Can you work these out from the model? Positions are in its coordinate system, mm. Give positions to 0.01 mm unless a question says otherwise; leave off trailing zeros. Order: outer loops, then holes, each group sorted by start corner. A loop starts at its lowest first (then second) coordinate and runs counter-clockwise, first axis right, second up. Notation, with made-up numbers: (48.5, 33.25) - (96.5, 33.25) arc R17 ccw to (96.5, 48.25) - close; hole circle Ø8 at (17.25, 11.25). An arc over 180 degrees is marked (long way). Answer as a JSON object with one key per item and string values.
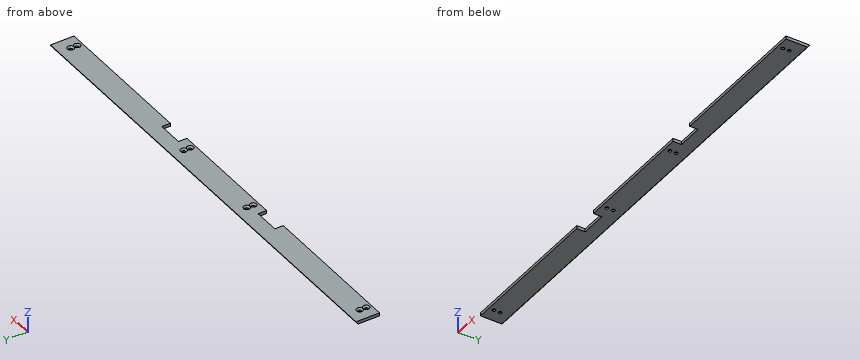
```python
from build123d import *

# Parameters (mm, degrees)
F0_W           = 1840
F0_H           = 92
F1_DEPTH       = 6
F2_W           = 100
F2_H           = 33
F3_DEPTH       = 12.001
F5_DEPTH       = 1840.001
F7_D           = 13
F7_CSINK_D     = 25
F7_CSINK_ANGLE = 90


with BuildPart() as f1:
    # F0 (on Top) → F1 (new body, symmetric)
    with BuildSketch(Plane.XY):
        Rectangle(F0_W, F0_H)
    extrude(amount=F1_DEPTH, both=True)

    # F2 (on face) → F3 (cut, through all)
    with BuildSketch(Plane.XY.offset(6)):
        with Locations((-290, -29.5)):
            Rectangle(F2_W, F2_H)
        with Locations((290, -29.5)):
            Rectangle(F2_W, F2_H)
    extrude(amount=-F3_DEPTH, mode=Mode.SUBTRACT)

    # F4 (on face) → F5 (cut, through all)
    with BuildSketch(Plane.YZ.offset(920)):
        Polygon((46, -6), (46, 4), (37.609004, -6), align=None)
    extrude(amount=-F5_DEPTH, mode=Mode.SUBTRACT)

    # F7 (through all)
    with Locations(Plane.XY.offset(6)):
        with Locations((-870, -1), (-870, -26), (-190, -1), (-190, -26), (190, -26), (190, -1), (870, -1), (870, -26)):
            CounterSinkHole(F7_D / 2, F7_CSINK_D / 2, counter_sink_angle=F7_CSINK_ANGLE)


solid = f1.part
```
Q1. I need wall thicknesses on L1, parallel to X at y = -40.5, z = 2.5; L2, parallel to X at y = -1, z = -4.4; L3, parallel to Y at x = 190, z = -2.45. Which ranges of each line are inside material? Lowest first, please.
Recorded:
{"L1": "x = -920 to -340, -240 to 240, 340 to 920", "L2": "x = -920 to -876.5, -863.5 to -196.5, -183.5 to 183.5, 196.5 to 863.5, 876.5 to 920", "L3": "y = -46 to -32.5, -19.5 to -7.5, 5.5 to 40.59"}
Q2. I'm going to push flat-ended pins straight in: pin 1 Ø10.5 at (x, y) = (-870, -1) entering from +Z; pin 2 Ø1.5 at (x, z) = (-132, 3.5) entering from +Y; pin 3 Ø3.5 at (x, z) = (269, -2) entering from -Y. Where does each tip first touch, or does it pass through?
Recorded:
{"pin 1": "passes through", "pin 2": "stops at y = 46", "pin 3": "stops at y = -13"}
Q3. If we section it at A-A, the plane z = -3.5: Count the separate pieces of the cut face and the enclosed holes in it, then the cut area to 3 significant figures.
Recorded:
{"separate pieces": "1", "enclosed holes": "8", "area": "150,000 mm^2"}
Q4. If we section it at B-B, the plane x = -322: Please give me the cut outline in (y, z), then the cut area to 3 significant figures.
Recorded:
{"outline": "(-13, -6) - (37.61, -6) - (46, 4) - (46, 6) - (-13, 6) - close", "area": "666 mm^2"}
